Model file for the job. Use its own axes, mm. Face numbers are marked on the shaded views. A direction names the side the tool comes from. Coordinates: 2 decimals unless noted, no trailing zeros. Write each loop counter-clockwise with the first axis right and the second up, starting at its lowest first coordinate (ties: lowest second). Pieces come first, ordered by that corner, then holes. Notation, with made-up numbers: M 17.25,50 L 31.25,50 A23 ccw 31.25,58 Z; hole C 30.5,17.5 d5. An arc over 180 degrees is marked long. One line per question, with ' | ' between items. Start each with the question number.
(1) Cut at A-A (x = 37). Write the cut outline in (y, z), plus the area to 3 significant figures.
(2) Tool access for the marked faces 1 and 2: list every direction of +Z, -Z, +X, -X, +Y, -Y with a clear straight run to the whole face (end or side of a thin tool).
(3) Cut at B-B (y = -4). Write the cut outline in (x, z).
(4) Cut at C-C (z = 12). Write the cut outline in (x, y), plus the area to 3 significant figures.
(5) Flat gauge pins, fed straight in: pin 1 Ø11 at (x, y) = (27.5, -12) entering from +Z (3 decimals); pin 2 Ø10 at (x, z) = (30, 29) entering from -Y; pin 3 Ø5 at (x, z) = (32.5, -4) entering from -Y. Where does each tip first touch, or does it go through?
(6) Wall check: probe 1 along Y at (x, z) = (28.5, -4.5); probe 2 along Y at (x, z) = (7, 37.5); probe 3 along Z at (x, y) = (16, -53). Give the ranges that are in metal, low to high.
from build123d import *

# Parameters (mm, degrees)
F0_W     = 18.416568
F0_H     = 22.800551
F1_DEPTH = 51.816


with BuildPart() as f1:
    # F0 (on Right) → F1 (new body)
    with BuildSketch(Plane.YZ):
        Polygon((42.630378, -34.009408), (42.630378, 41.846275), (-2.095759, 41.846275), (-2.095759, 22.115029), (-2.095759, -34.009408), align=None)
        Polygon((-2.095759, -34.009408), (-2.095759, 22.115029), (-24.020061, 22.115029), (-24.020061, 5.891558), (-24.020061, -34.009408), align=None)
        Polygon((-43.752097, -34.009408), (-24.020061, -34.009408), (-24.020061, 5.891558), (-43.752097, 5.891558), (-43.752097, -11.208857), align=None)
        with Locations((-52.960381, -22.609133)):
            Rectangle(F0_W, F0_H)
    extrude(amount=F1_DEPTH)


solid = f1.part
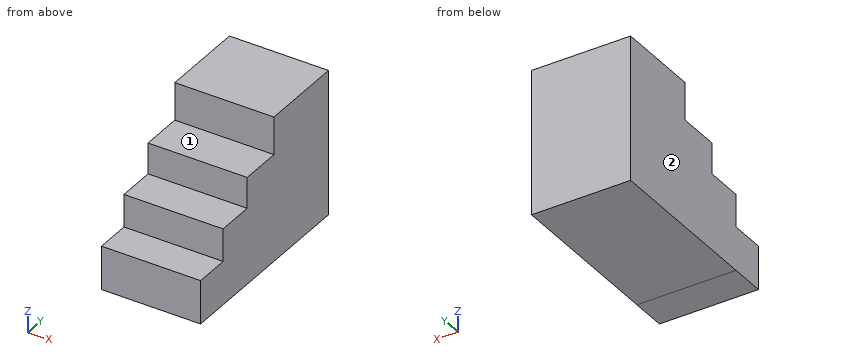
Filled in:
1) outline: M -62.17,-34.01 L 42.63,-34.01 L 42.63,41.85 L -2.1,41.85 L -2.1,22.12 L -24.02,22.12 L -24.02,5.89 L -43.75,5.89 L -43.75,-11.21 L -62.17,-11.21 Z | area: 5,830 mm²
2) face 1: +Z, +X, -X, -Y | face 2: +Z, -Z, -X, +Y, -Y
3) outline: M 0,-34.01 L 51.82,-34.01 L 51.82,22.12 L 0,22.12 Z
4) outline: M 0,-24.02 L 51.82,-24.02 L 51.82,42.63 L 0,42.63 Z | area: 3,450 mm²
5) pin 1: z = 22.115 | pin 2: y = -2.1 | pin 3: y = -43.75
6) probe 1: -43.75 to 42.63 | probe 2: -2.1 to 42.63 | probe 3: -34.01 to -11.21
